Source: CAD feature listing. Evaluate the final solid. Frame: model axes, mm. Give positions to 0.01 mm unless a question says otherwise; leave off trailing zeros. Write each loop counter-clockwise with the first axis right and the second up, starting at its lowest first coordinate (ties: lowest second). Pieces come first, ordered by that corner, then holes. Notation, with made-up numbers: (70.25, 60.25) -> (84.25, 60.25) arc R32 cw to (84.25, 98.25) -> close; hole circle Ø7 at (45.5, -35.5). An arc over 180 degrees is marked (long way). Use one line per item in the form item = value. Start each with the question number.
(1) Cut plane A-A, the plane x = 3.25. Output: boundary loops of the cut face in (y, z), and give its area (3 significant figures).
(2) Cut plane D-D, the plane z = 7.5. Output: boundary loops of the cut face in (x, y), and give its area (3 significant figures).
(3) Cut plane C-C, the plane x = 15.5. Output: boundary loops of the cut face in (y, z), and give its area (3 significant figures).
(4) Draft query along Y for faces 1 (the face through (23, -3, 5)), 2 (the face through (6.71, 6.86, 7.47)), 3 (the face through (4, 5, 5.5)). Return one class per face: pulls with the +Y half, pulls with the -Y half, needs draft (parallel to the pull), parting line crosses it, or undercut.
(5) First-contact query: P1, Ø4, axis at x = 23.5, y = 8.5, coming from the -Z side; P2, Ø1, axis at x = 39, z = 7.5, coming from the +Y side; P3, Ø12, axis at x = 20, y = 43.5, coming from the +Z side; P4, Ø6, axis at y = 17, z = 7, coming from the +X side. Flat tips, straight axial feed; report the tip coordinate or a pass-through.
(6) Material intervals for line 1 along Y through (x, z) = (3.25, 7.75); line 2 along X through (y, z) = (3.25, 0.6), sorted ascending. Write a range as from..to.
Autodesk Fusion 360 part; units mm, degrees
sketch "Sketch1" plane through (0, 0, 0) normal (0, 0, 1) x (1, 0, 0)
  line L0 (0, 0) -> (50, 0)
  line L1 (50, 0) -> (50, 50)
  line L2 (50, 50) -> (0, 50)
  line L3 (0, 50) -> (0, 0)
  dimension "d1" = 50
  dimension "d2" = 50
extrude "Extrude1" add sketch "Sketch1" along normal blind 3
sketch "Sketch2" plane through (0, 0, 0) normal (0, 0, 1) x (1, 0, 0)
  line L0 (50, 50) -> (0, 50)
  line L1 (50, 0) -> (50, 50)
  line L2 (0, 0) -> (50, 0)
  line L3 (0, 50) -> (0, 0)
  line L4 (-3, 50) -> (-3, -3)
  line L5 (-3, -3) -> (50, -3)
  line L6 (-3, 50) -> (0, 50)
  line L7 (50, 0) -> (50, -3)
  dimension "d8" = 3
extrude "Extrude2" add sketch "Sketch2" along normal blind 10 contours L2 L3 L4 L5 L6 L7
ref_plane "WorkPlane1" through (25, 25, 5.5) normal (0, 0, 1) x (1, 0, 0)
sketch "Sketch4" plane through (0, 0, 5.5) normal (0, 0, 1) x (1, 0, 0)
  circle A0 centre (3.25, 3.25) radius 5
  line L0 (0, 0) -> (0, 50)
  line L1 (50, 0) -> (0, 0)
  dimension "d15" = 3.25
  dimension "d16" = 3.25
  dimension "d25" = 10
extrude "Extrude3" add sketch "Sketch4" along normal blind 4.5 contours A0 L0 L1 picked at (4.5229, 4.5125)
sketch "Sketch5" plane through (0, 0, 10) normal (0, 0, 1) x (-1, 0, 0)
  line L0 (3, -50) -> (3, 3)
  line L1 (3, 3) -> (-50, 3)
  line L2 (-50, 3) -> (-50, 0)
  line L3 (-50, 0) -> (-7.0497, 0)
  arc A0 (-7.0497, 0) -> (0, -7.0497) centre (-3.25, -3.25) ccw
  line L4 (0, -7.0497) -> (0, -50)
  line L5 (0, -50) -> (3, -50)
hole "Hole2" at (3.25, 3.25, 10) direction (0, 0, -1) diameter 3 end up to surface (10 mm away)
fillet "Fillet1" radius 0.5 12 edges at (23.5, -3, 0) (50, -3, 5) (23.5, -3, 10) (-3, -3, 5) (-3, 23.5, 0) (-3, 23.5, 10) (23.5, 50, 0) (50, 23.5, 0) (-1.5, 50, 10) (-3, 50, 5) (50, -1.5, 10) (50, 50, 1.5)
fillet "Fillet2" radius 0.5 10 edges at (50, 0, 6.25) (49.8536, 0, 9.8536) (28.2748, 0, 10) (0, 28.2748, 10) (0, 49.8536, 9.8536) (0, 50, 6.25) (50, 24.75, 3) (49.8536, 49.8536, 3) (24.75, 50, 3) (6.7855, 6.7855, 10)
equation "d16 = d15"
equation "d17 = 7 mm - 2.5 mm"
Geometry says:
q1.outline = (-3, 0.5) arc R0.5 ccw to (-2.5, 0) -> (1.75, 0) -> (1.75, 3) -> (0, 3) -> (0, 5.5) -> (1.75, 5.5) -> (1.75, 10) -> (-2.5, 10) arc R0.5 ccw to (-3, 9.5) -> close; (4.75, 0) -> (49.5, 0) arc R0.5 ccw to (50, 0.5) -> (50, 2.5) arc R0.5 ccw to (49.5, 3) -> (4.75, 3) -> close; (4.75, 5.5) -> (8.25, 5.5) -> (8.25, 9.5) arc R0.5 ccw to (7.75, 10) -> (4.75, 10) -> close
q1.area = 194 mm^2
q2.outline = (-3, -2.5) arc R0.5 ccw to (-2.5, -3) -> (49.5, -3) arc R0.5 ccw to (50, -2.5) -> (50, -0.5) arc R0.5 ccw to (49.5, 0) -> (7.05, 0) arc R5 ccw to (0, 7.05) -> (0, 49.5) arc R0.5 ccw to (-0.5, 50) -> (-2.5, 50) arc R0.5 ccw to (-3, 49.5) -> close; hole circle Ø3 at (3.25, 3.25)
q2.area = 362 mm^2
q3.outline = (-3, 0.5) arc R0.5 ccw to (-2.5, 0) -> (49.5, 0) arc R0.5 ccw to (50, 0.5) -> (50, 2.5) arc R0.5 ccw to (49.5, 3) -> (0, 3) -> (0, 9.5) arc R0.5 ccw to (-0.5, 10) -> (-2.5, 10) arc R0.5 ccw to (-3, 9.5) -> close
q3.area = 180 mm^2
q4.face_1 = pulls with the -Y half
q4.face_2 = undercut
q4.face_3 = needs draft
q5.P1 = 0
q5.P2 = 0
q5.P3 = 3
q5.P4 = 0
q6.line_1 = -3..1.75, 4.75..8.25
q6.line_2 = -3..1.75, 4.75..50
